Drawing for the job (mm, zero at the part's lowest x, y, z). A direction names the side the tool comes from. Coordinates: 2 decimals unless noted, no trailing zeros. Order: outer loops, then holes, each group sorted by start corner. A loop starts at its lowest first (then second) coordinate and runs counter-clockwise, first axis right, second up. Notation, with made-up numbers: M -35,-17.5 L -13,-17.5 A15 cw -13,-3.5 Z; hole C 7.25,54.5 d9. An arc over 180 degrees is marked long. Write item = value, one per line. Start each with the question number.
Q1. Pin check, flat tips, straight feed: P1, Ø3, axis at y = 5, z = 17, coming from the +X side; P2, Ø4, axis at x = 8.5, y = 3, coming from the -Z side; P3, Ø4, axis at y = 6.5, z = 10.5, coming from the +X side. Stop position of each tip, or through.
Q2. Band-saw the part on D-D on y = 7.25. Write the cut outline in (x, z).
Q3. Band-saw the part on A-A on x = 13. Write the cut outline in (y, z), plus the area to 3 significant figures.
Q4. Band-saw the part on B-B on z = 13. Write the cut outline in (x, y), plus the area to 3 significant figures.
Q5. Band-saw the part on C-C on y = 5.25. Write the cut outline in (x, z).
Q6. Drill centre lines: probe 1 along Y at (x, z) = (14.5, 21.5); probe 2 along Z at (x, y) = (12.75, 1); probe 3 along Z at (x, y) = (7.5, 3.25). Where is each one in solid material? Low to high.
Q7. 3-axis set-ups, long thin cutter, end or side, ignore diameter. For the marked faces 1 and 2: which of +Z, -Z, +X, -X, +Y, -Y reach the whole face in a straight line?
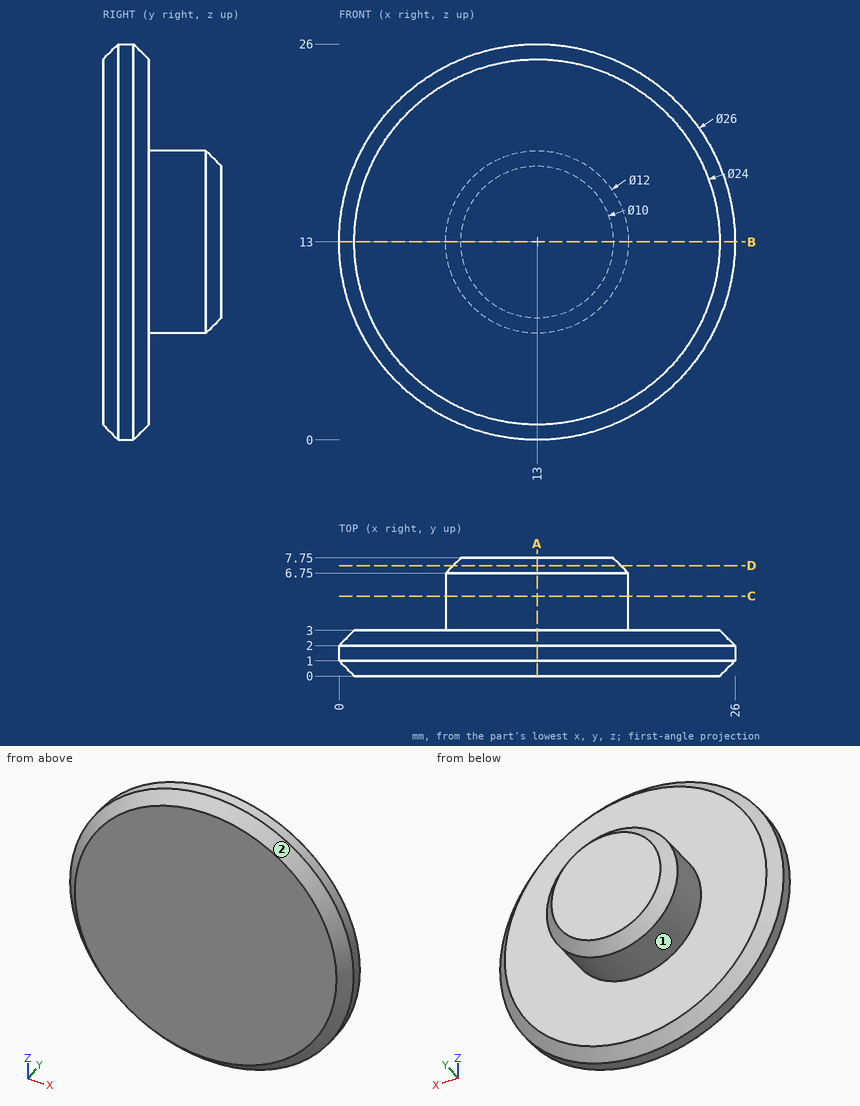
Recorded:
q1.P1 = 18.45
q1.P2 = 0.3
q1.P3 = 18.98
q2.outline = C 13,13 d11
q3.outline = M 0,1 L 1,0 L 2,0 L 3,1 L 3,7 L 6.75,7 L 7.75,8 L 7.75,18 L 6.75,19 L 3,19 L 3,25 L 2,26 L 1,26 L 0,25 Z
q3.area = 132 mm2
q4.outline = M 0,1 L 1,0 L 25,0 L 26,1 L 26,2 L 25,3 L 19,3 L 19,6.75 L 18,7.75 L 8,7.75 L 7,6.75 L 7,3 L 1,3 L 0,2 Z
q4.area = 132 mm2
q5.outline = C 13,13 d12
q6.probe_1 = 0 to 3
q6.probe_2 = 0 to 26
q6.probe_3 = 10.6 to 15.4
q7.face_1 = +Y
q7.face_2 = -Y
